```python
from build123d import *

# Parameters (mm, degrees)
SKETCH1_W          = 9.95
SKETCH1_H          = 0.5
SKETCH1_W_2        = 2.8
SKETCH1_H_2        = 1.2
CUT_EXTRUDE2_START = 2
CUT_EXTRUDE2_DEPTH = 2
SKETCH3_W          = 1.17
SKETCH3_H          = 1.465
SKETCH3_H_2        = 1.17
SKETCH3_W_2        = 1.465
CUT_EXTRUDE3_DEPTH = 4.3
FILLET1_R          = 0.3
FILLET2_R          = 1
FILLET3_R          = 2


with BuildPart() as part:
    # Sketch1 → Revolve1 (revolve)
    with BuildSketch(Plane(origin=(0, 0, 0), x_dir=(1, 0, 0), z_dir=(0, 1, 0)), mode=Mode.PRIVATE) as revolve1_sk:
        with BuildLine():
            Line((2.8, 0), (0, 0))
            Line((0, 0), (0, -4.5))
            ThreePointArc((0, -4.5), (6.130099918, -4.625052018), (12.25, -5))
            Line((12.25, -5), (14.25, -5))
            Line((14.25, -5), (14.25, 0))
            Line((14.25, 0), (12.75, 0))
            Line((12.75, 0), (12.75, -3.1))
            Line((12.75, -3.1), (12.75, -3.6))
            Line((12.75, -3.6), (2.8, -3.6))
            Line((2.8, -3.6), (2.8, -3.1))
            Line((2.8, -3.1), (2.8, 0))
        make_face()
        with Locations((7.775, -3.35)):
            Rectangle(SKETCH1_W, SKETCH1_H)
        with Locations((1.4, 0.6)):
            Rectangle(SKETCH1_W_2, SKETCH1_H_2)
    revolve(revolve1_sk.sketch.rotate(Axis((0, 0, 0), (0, 0, 1)), 180), axis=Axis((0, 0, 0), (0, 0, 1)))

    # Sketch2 → Cut-Extrude2 (cut)
    with BuildSketch(Plane.XY.offset(CUT_EXTRUDE2_START)):
        with BuildLine():
            Line((10.747952079, 9.404591185), (9.404591185, 10.747952079))
            Line((9.404591185, 10.747952079), (6.858864783, 10.747952079))
            ThreePointArc((6.858864783, 10.747952079), (9.01561146, 9.01561146), (10.747952079, 6.858864783))
            Line((10.747952079, 6.858864783), (10.747952079, 9.404591185))
        make_face()
        Polygon((9.404591185, 10.747952079), (8.131727984, 12.02081528), (6.858864783, 10.747952079), align=None)
        Polygon((12.02081528, 8.131727984), (10.747952079, 9.404591185), (10.747952079, 6.858864783), align=None)
        Polygon((12.02081528, -8.131727984), (10.747952079, -6.858864783), (10.747952079, -9.404591185), align=None)
        with BuildLine():
            Line((10.747952079, -9.404591185), (10.747952079, -6.858864783))
            ThreePointArc((10.747952079, -6.858864783), (9.01561146, -9.01561146), (6.858864783, -10.747952079))
            Line((6.858864783, -10.747952079), (9.404591185, -10.747952079))
            Line((9.404591185, -10.747952079), (10.747952079, -9.404591185))
        make_face()
        Polygon((9.404591185, -10.747952079), (6.858864783, -10.747952079), (8.131727984, -12.02081528), align=None)
        Polygon((-8.131727984, -12.02081528), (-6.858864783, -10.747952079), (-9.404591185, -10.747952079), align=None)
        with BuildLine():
            ThreePointArc((-6.858864783, -10.747952079), (-9.01561146, -9.01561146), (-10.747952079, -6.858864783))
            Line((-10.747952079, -6.858864783), (-10.747952079, -9.404591185))
            Line((-10.747952079, -9.404591185), (-9.404591185, -10.747952079))
            Line((-9.404591185, -10.747952079), (-6.858864783, -10.747952079))
        make_face()
        Polygon((-10.747952079, -9.404591185), (-10.747952079, -6.858864783), (-12.02081528, -8.131727984), align=None)
        Polygon((-12.02081528, 8.131727984), (-10.747952079, 6.858864783), (-10.747952079, 9.404591185), align=None)
        with BuildLine():
            ThreePointArc((-10.747952079, 6.858864783), (-9.01561146, 9.01561146), (-6.858864783, 10.747952079))
            Line((-6.858864783, 10.747952079), (-9.404591185, 10.747952079))
            Line((-9.404591185, 10.747952079), (-10.747952079, 9.404591185))
            Line((-10.747952079, 9.404591185), (-10.747952079, 6.858864783))
        make_face()
        Polygon((-9.404591185, 10.747952079), (-6.858864783, 10.747952079), (-8.131727984, 12.02081528), align=None)
    extrude(amount=-CUT_EXTRUDE2_DEPTH, mode=Mode.SUBTRACT)

    # Sketch3 → Cut-Extrude3 (cut)
    with BuildSketch(Plane(origin=(0, 0, -1.2), x_dir=(-1, 0, 0), z_dir=(0, 0, -1))):
        with Locations((0, 1.3175)):
            Rectangle(SKETCH3_W, SKETCH3_H)
        Rectangle(SKETCH3_W, SKETCH3_H_2)
        with Locations((0, -1.3175)):
            Rectangle(SKETCH3_W, SKETCH3_H)
        with Locations((-1.3175, 0)):
            Rectangle(SKETCH3_W_2, SKETCH3_H_2)
        with Locations((1.3175, 0)):
            Rectangle(SKETCH3_W_2, SKETCH3_H_2)
    extrude(amount=-CUT_EXTRUDE3_DEPTH, mode=Mode.SUBTRACT)

    # Fillet1
    fillet1_edges = [part.edges().sort_by_distance(p)[0] for p in [
        (0.585, 0.585, 0.95),
        (0.585, -0.585, 0.95),
        (-0.585, -0.585, 0.95),
        (-0.585, 0.585, 0.95),
    ]]
    fillet(fillet1_edges, radius=FILLET1_R)

    # Fillet2
    fillet2_edges = [part.edges().sort_by_distance(p)[0] for p in [
        (12.75, 0, 3.1),
    ]]
    fillet(fillet2_edges, radius=FILLET2_R)

    # Fillet3
    fillet3_edges = [part.edges().sort_by_distance(p)[0] for p in [
        (14.25, 0, 5),
    ]]
    fillet(fillet3_edges, radius=FILLET3_R - 0.0001)  # a hair under: the kernel refuses the full size


solid = part.part
```
Check sheet for the modelled part. Datum: model origin and axes. Units: mm. A direction names the side the tool comes from. Coordinates: 2 decimals unless noted, no trailing zeros. Order: outer loops, then holes, each group sorted by start corner. A loop starts at its lowest first (then second) coordinate and runs counter-clockwise, first axis right, second up. Notation, with made-up numbers: (20.25, -22) -> (72.25, -22) arc R24 ccw to (72.25, 6) -> close; hole circle Ø9 at (72.5, 66.25). An arc over 180 degrees is marked (long way). Write each question's results on one line, items separated by ' | '. Start each with the question number.
1) Material ranges on line 1 along Y through (x, z) = (0, 1.6); line 2 along X through (y, z) = (0.25, 2); line 3 along Y through (x, z) = (-1.25, 1) (1 decimal), recorded low to high.
2) Depth check by flat-ended pin: pin 1 (3 mm diameter, centred on x = 3.5, y = -13, fed in from -Z); pin 2 (1.3 mm diameter, centred on y = -1.5, z = 2, fed in from +X); pin 3 (2 mm diameter, centred on y = 5, z = 2.5, fed in from -X). Enter the tip coordinate at first touch or a pass-through.
3) Set-up check for faces 1 (the face through (-13, 0, 0)), 2 (the face through (0, 13, 0)), 3 (the face through (0.585, 1.5, 0.9)): record each of +Z, -Z, +X, -X, +Y, -Y from which the full face is reachable in a straight line by a thin tool's end or side.
4) Draft check along Y on faces 4 (the face through (1.5, 0.585, 0.9)), 5 (the face through (2.4, 2.4, 3.1)), 6 (the face through (-11.28, -7.39, 1.01)), 7 (the face through (11.28, 7.39, 1.01)). Enter one of: pulls with the +Y half, pulls with the -Y half, needs draft (parallel to the pull), parting line crosses it, or undercut.
5) Section check B-B (z = -0.5). Enter the section's corners in (x, y) (3 decimals).
6) Section check A-A (z = 1). Count the separate pieces of the cut face and the enclosed holes in it, and give its area (3 significant figures).
Checked values:
1) line 1: -14.25 to -12.75, -2.8 to -2.05, 2.05 to 2.8, 12.75 to 14.25 | line 2: -14.25 to -12.75, -2.79 to -2.05, 2.05 to 2.79, 12.75 to 14.25 | line 3: -14.2 to -12.7, -2.5 to -0.6, 0.6 to 2.5, 12.7 to 14.2
2) pin 1: z = 0 | pin 2: x = 14.22 | pin 3: x = -13.68
3) face 1: -Z, -X, +Y, -Y | face 2: -Z, +X, -X, +Y | face 3: -Z
4) face 4: undercut | face 5: undercut | face 6: pulls with the -Y half | face 7: pulls with the +Y half
5) outline: circle Ø5.6 at (0, 0); hole (-2.05, -0.585) -> (-0.885, -0.585) arc R0.3 cw to (-0.585, -0.885) -> (-0.585, -2.05) -> (0.585, -2.05) -> (0.585, -0.885) arc R0.3 cw to (0.885, -0.585) -> (2.05, -0.585) -> (2.05, 0.585) -> (0.885, 0.585) arc R0.3 cw to (0.585, 0.885) -> (0.585, 2.05) -> (-0.585, 2.05) -> (-0.585, 0.885) arc R0.3 cw to (-0.885, 0.585) -> (-2.05, 0.585) -> close
6) separate pieces: 5 | enclosed holes: 1 | area: 110 mm²
